Read the model definition and answer for the solid it produces. Units are mm, in the model's axes. Round coordinates to 2 decimals unless told otherwise and drop trailing zeros. Loops run counter-clockwise (first coordinate to the right, second up) from the corner with the lowest first, then second, coordinate; pieces in that order, holes last. Notation, with made-up numbers: M 4.5,69.5 L 28.5,69.5 A5 cw 28.5,73.5 Z; hole C 88,43 d9. An arc over 180 degrees is marked long. Write each question's results on one line, items separated by ' | '.
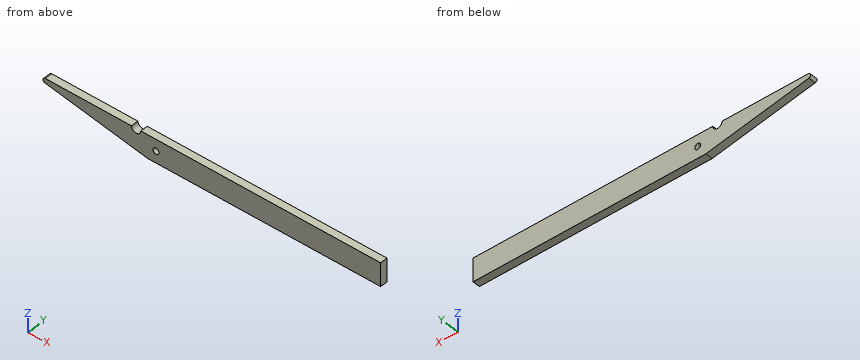
from build123d import *

# Parameters (mm, degrees)
BOSS_EXTRUDE1_DEPTH = 3.175
CUT_EXTRUDE1_REACH  = 227.249
SKETCH2_R           = 1.27
CUT_EXTRUDE2_DEPTH  = 226.248510263
SKETCH4_W           = 85
SKETCH4_H           = 10
CUT_EXTRUDE3_DEPTH  = 226.248510263


with BuildPart() as part:
    # Sketch1 → Boss-Extrude1 (new body)
    with BuildSketch(Plane(origin=(0, 0, 0), x_dir=(1, 0, 0), z_dir=(0, 1, 0))):
        with BuildLine():
            Line((0, 0), (-224.004023854, 0))
            ThreePointArc((-224.004023854, 0), (-225, 0.910381269), (-224.18254009, 1.983936966))
            Line((-224.18254009, 1.983936966), (-180, 10))
            Line((-180, 10), (0, 10))
            ThreePointArc((0, 10), (5, 5), (0, 0))
        make_face()
    extrude(amount=BOSS_EXTRUDE1_DEPTH)

    # Sketch2 → Cut-Extrude1 (cut, up to next)
    with BuildSketch(Plane(origin=(0, 3.175, 0), x_dir=(1, 0, 0), z_dir=(0, 1, 0)), mode=Mode.PRIVATE) as cut_extrude1_sk1:
        with Locations(Location((-50, 5, 0), (0, 0, 270))):
            Circle(SKETCH2_R)
    cut_extrude1_tool1 = extrude(cut_extrude1_sk1.sketch, amount=-CUT_EXTRUDE1_REACH, mode=Mode.PRIVATE) & part.part
    # Sketch2 → Cut-Extrude1 (cut, up to next)
    with BuildSketch(Plane(origin=(0, 3.175, 0), x_dir=(1, 0, 0), z_dir=(0, 1, 0)), mode=Mode.PRIVATE) as cut_extrude1_sk2:
        with Locations(Location((0, 5, 0), (0, 0, 270))):
            Circle(SKETCH2_R)
    cut_extrude1_tool2 = extrude(cut_extrude1_sk2.sketch, amount=-CUT_EXTRUDE1_REACH, mode=Mode.PRIVATE) & part.part
    # Sketch2 → Cut-Extrude1 (cut, up to next)
    with BuildSketch(Plane(origin=(0, 3.175, 0), x_dir=(1, 0, 0), z_dir=(0, 1, 0)), mode=Mode.PRIVATE) as cut_extrude1_sk3:
        with Locations(Location((-176.52, 5, 0), (0, 0, 270))):
            Circle(SKETCH2_R)
    cut_extrude1_tool3 = extrude(cut_extrude1_sk3.sketch, amount=-CUT_EXTRUDE1_REACH, mode=Mode.PRIVATE) & part.part
    add(cut_extrude1_tool1.solids().sort_by_distance((-50, 3.175, -5))[0], mode=Mode.SUBTRACT)
    add(cut_extrude1_tool2.solids().sort_by_distance((0, 3.175, -5))[0], mode=Mode.SUBTRACT)
    add(cut_extrude1_tool3.solids().sort_by_distance((-176.52, 3.175, -5))[0], mode=Mode.SUBTRACT)

    # Sketch3 → Cut-Extrude2 (cut, through all)
    with BuildSketch(Plane(origin=(0, 3.175, 0), x_dir=(1, 0, 0), z_dir=(0, 1, 0))):
        with BuildLine():
            Line((-187, 0), (-183, 0))
            ThreePointArc((-183, 0), (-185, 2), (-187, 0))
        make_face()
    extrude(amount=-CUT_EXTRUDE2_DEPTH, mode=Mode.SUBTRACT)

    # Sketch4 → Cut-Extrude3 (cut, through all)
    with BuildSketch(Plane.XZ):
        with Locations((-37.5, -5)):
            Rectangle(SKETCH4_W, SKETCH4_H)
    extrude(amount=-CUT_EXTRUDE3_DEPTH, mode=Mode.SUBTRACT)


solid = part.part
Item 1: The part is cut by section D-D (x = -199). Determine the outline of the cut face in (y, z) (3 decimals).
Outcome:
outline: M 0,-6.553 L 3.175,-6.553 L 3.175,0 L 0,0 Z
Item 2: The part is cut by section C-C (y = 1.05). Determine the outline of the cut face in (x, z), plus the area to 3 significant figures.
Outcome:
outline: M -224.18,-1.98 L -180,-10 L -80,-10 L -80,0 L -183,0 A2 cw -187,0 L -224,0 A1 ccw Z; hole C -176.52,-5 d2.54 | area: 1,250 mm2
Item 3: Straight lines are drawn through the part: line 1 (Z direction, x = -176.52, y = 1.55); line 2 (X direction, y = 2, z = -0.25); line 3 (X direction, y = 1.6, z = -1.5). For each, find the intervals that lie inside material, in ascending order.
Outcome:
line 1: z = -10 to -6.27, -3.73 to 0 | line 2: x = -224.67 to -186.98, -183.02 to -80 | line 3: x = -224.87 to -186.32, -183.68 to -80
Item 4: A flat-ended cylindrical pin translates along its axis: pin 1 (4 mm diameter, centred on x = -201.5, z = -2, fed in from -Y). Find the tip coordinate at first contact, or state that the pin passes through.
Outcome:
pin 1: stops at y = 0
Item 5: The part is cut by section A-A (x = -176.52). Determine the outline of the cut face in (y, z) (3 decimals), plus the area to 3 significant figures.
Outcome:
outline: M 0,-10 L 3.175,-10 L 3.175,-6.27 L 0,-6.27 Z; M 0,-3.73 L 3.175,-3.73 L 3.175,0 L 0,0 Z | area: 23.7 mm2
Item 6: The part is cut by section B-B (z = -5). Determine the outline of the cut face in (x, y) (3 decimals).
Outcome:
outline: M -207.559,0 L -177.79,0 L -177.79,3.175 L -207.559,3.175 Z; M -175.25,0 L -80,0 L -80,3.175 L -175.25,3.175 Z
